```python
from build123d import *

# Parameters (mm, degrees)
BOSS_EXTRUDE1_DEPTH        = 40
BOSS_EXTRUDE2_DEPTH        = 30
BOSS_EXTRUDE3_DEPTH        = 5
SKETCH1_6_R                = 5
BOSS_EXTRUDE4_DEPTH        = 15
F_10_0_10_DIAMETER_HOLE1_D = 10
FILLET2_R                  = 20


with BuildPart() as part:
    # Sketch1 → Boss-Extrude1 (new, symmetric)
    with BuildSketch(Plane.XY):
        with BuildLine():
            ThreePointArc((-31.224989992, 25), (-37.742546282, 13.247648854), (-40, 0))
            Line((-40, 0), (-25, 0))
            ThreePointArc((-25, 0), (0, 25), (25, 0))
            Line((25, 0), (40, 0))
            ThreePointArc((40, 0), (37.742546282, 13.247648854), (31.224989992, 25))
            ThreePointArc((31.224989992, 25), (26.062179457, 30.344073589), (20, 34.641016151))
            ThreePointArc((20, 34.641016151), (0, 40), (-20, 34.641016151))
            ThreePointArc((-20, 34.641016151), (-26.062179457, 30.344073589), (-31.224989992, 25))
        make_face()
    extrude(amount=BOSS_EXTRUDE1_DEPTH, both=True)

    # Sketch1_3 → Boss-Extrude2 (add, symmetric)
    with BuildSketch(Plane.XY):
        with BuildLine():
            ThreePointArc((31.224989992, 25), (37.742546282, 13.247648854), (40, 0))
            Line((40, 0), (80, 0))
            Line((80, 0), (80, 25))
            Line((80, 25), (45, 25))
            Line((45, 25), (31.224989992, 25))
        make_face()
        with BuildLine():
            Line((-80, 25), (-80, 0))
            Line((-80, 0), (-40, 0))
            ThreePointArc((-40, 0), (-37.742546282, 13.247648854), (-31.224989992, 25))
            Line((-31.224989992, 25), (-45, 25))
            Line((-45, 25), (-80, 25))
        make_face()
    extrude(amount=BOSS_EXTRUDE2_DEPTH, both=True)

    # Sketch1_5 → Boss-Extrude3 (add, symmetric)
    with BuildSketch(Plane.XY):
        with BuildLine():
            Line((20, 50), (20, 34.641016151))
            ThreePointArc((20, 34.641016151), (26.062179457, 30.344073589), (31.224989992, 25))
            Line((31.224989992, 25), (45, 25))
            Line((45, 25), (20, 50))
        make_face()
        with BuildLine():
            Line((-45, 25), (-31.224989992, 25))
            ThreePointArc((-31.224989992, 25), (-26.062179457, 30.344073589), (-20, 34.641016151))
            Line((-20, 34.641016151), (-20, 50))
            Line((-20, 50), (-45, 25))
        make_face()
    extrude(amount=BOSS_EXTRUDE3_DEPTH, both=True)

    # Sketch1_6 → Boss-Extrude4 (add, symmetric)
    with BuildSketch(Plane.XY):
        with BuildLine():
            Line((-20, 50), (-20, 34.641016151))
            ThreePointArc((-20, 34.641016151), (0, 40), (20, 34.641016151))
            Line((20, 34.641016151), (20, 50))
            ThreePointArc((20, 50), (0, 70), (-20, 50))
        make_face()
        with Locations((0, 50)):
            Circle(SKETCH1_6_R, mode=Mode.SUBTRACT)
    extrude(amount=BOSS_EXTRUDE4_DEPTH, both=True)

    # 10.0 _10_ Diameter Hole1 (through all)
    with Locations(Plane(origin=(-60, 25, -10), x_dir=(1, 0, 0), z_dir=(0, 1, 0))):
        with Locations((0, 0), (0, -20), (120, -20), (120, 0)):
            Hole(F_10_0_10_DIAMETER_HOLE1_D / 2)

    # Fillet2
    fillet2_edges = [part.edges().sort_by_distance(p)[0] for p in [
        (80, 12.5, -30),
        (80, 12.5, 30),
        (-80, 12.5, 30),
        (-80, 12.5, -30),
    ]]
    fillet(fillet2_edges, radius=FILLET2_R)


solid = part.part
```
Verification items for the finished model (mm, model axes). A direction names the side the tool comes from. Coordinates: 2 decimals unless noted, no trailing zeros. Loops run counter-clockwise (first coordinate to the right, second up) from the corner with the lowest first, then second, coordinate; pieces in that order, holes last. Notation, with made-up numbers: (11.25, 64.5) - (51.25, 64.5) arc R16 cw to (51.25, 75.5) - close; hole circle Ø4 at (24, 38). An arc over 180 degrees is marked (long way). Return JSON: item names as keys, results as strings.
1. Go/stop test with flat-tipped pins: pin 1 (6 mm diameter, centred on y = 16, z = -29.5, fed in from +X); pin 2 (11.5 mm diameter, centred on x = 0, y = 50, fed in from +Z); pin 3 (6 mm diameter, centred on x = 0.5, z = 6, fed in from +Y). Record where each tip stops, or that it passes through.
Established:
{"pin 1": "stops at x = 71.3", "pin 2": "stops at z = 15", "pin 3": "stops at y = 70"}
2. Section check D-D, the plane y = 62.5. Record the boundary of the cut face in (x, z).
Established:
{"outline": "(-15.61, -15) - (15.61, -15) - (15.61, 15) - (-15.61, 15) - close"}
3. Mould release check, pull along X, two halves, no side actions. Record for faces 1 (the cylindrical face through (65, 12, 10)), 2 (the flat face through (56, 25, 0)), 3 (the flat face through (-80, 13, 0)): +X half, -X half, draft (parallel to the pull), parting line (faces both ways), or undercut.
Established:
{"face 1": "undercut", "face 2": "draft", "face 3": "-X half"}
4. Section check C-C, the plane z = 26.5. Record the boundary of the cut face in (x, y).
Established:
{"outline": "(-71.3, 0) - (-25, 0) arc R25 cw to (25, 0) - (71.3, 0) - (71.3, 25) - (31.22, 25) arc R40 ccw to (-31.22, 25) - (-71.3, 25) - close"}
5. Section check A-A, the plane z = 8. Record the boundary of the cut face in (x, y), then the cut area to 3 significant figures.
Established:
{"outline": "(-80, 0) - (-64.58, 0) - (-64.58, 25) - (-80, 25) - close; (-55.42, 0) - (-25, 0) arc R25 cw to (25, 0) - (55.42, 0) - (55.42, 25) - (31.22, 25) arc R40 ccw to (20, 34.64) - (20, 50) arc R20 ccw to (-20, 50) - (-20, 34.64) arc R40 ccw to (-31.22, 25) - (-55.42, 25) - close; (64.58, 0) - (80, 0) - (80, 25) - (64.58, 25) - close; hole circle Ø10 at (0, 50)", "area": "4,230 mm2"}
6. Thickness scan on L1, parallel to Z at x = 58, y = 10; L2, parallel to Z at x = -13.5, y = 39.5; L3, parallel to Z at x = -33.5, y = 33.5. Record the ranges inside material, lowest first.
Established:
{"L1": "z = -30 to -14.58, -5.42 to 5.42, 14.58 to 30", "L2": "z = -15 to 15", "L3": "z = -5 to 5"}
7. Tool access check on faces 4 (the flat face through (-49, 13, -30)), 5 (the flat face through (49, 13, -30)), 6 (the flat face through (-49, 13, 30)), 7 (the flat face through (28, 35, 5)). Record the directions out of +Z, -Z, +X, -X, +Y, -Y that give a thin tool (end or side, any length) a straight path to the whole face; none if there is none.
Established:
{"face 4": "-Z, -X, +Y", "face 5": "-Z, +X, +Y", "face 6": "+Z, -X, +Y", "face 7": "+Z, +X, +Y"}
8. Section check B-B, the plane x = 43. Record the boundary of the cut face in (y, z).
Established:
{"outline": "(0, -30) - (25, -30) - (25, -5) - (27, -5) - (27, 5) - (25, 5) - (25, 30) - (0, 30) - close"}
